Build history of the part. All positions in model axes, mm. Give positions to 0.01 mm unless a question says otherwise; leave off trailing zeros. Order: outer loops, then holes, each group sorted by start corner. A loop starts at its lowest first (then second) coordinate and runs counter-clockwise, first axis right, second up. Notation, with made-up numbers: M -15.75,73.5 L 7.25,73.5 A19 cw 7.25,82.5 Z; hole C 15,69 d10. An arc over 180 degrees is marked long. One line per item, written item: value. Start each with the question number.
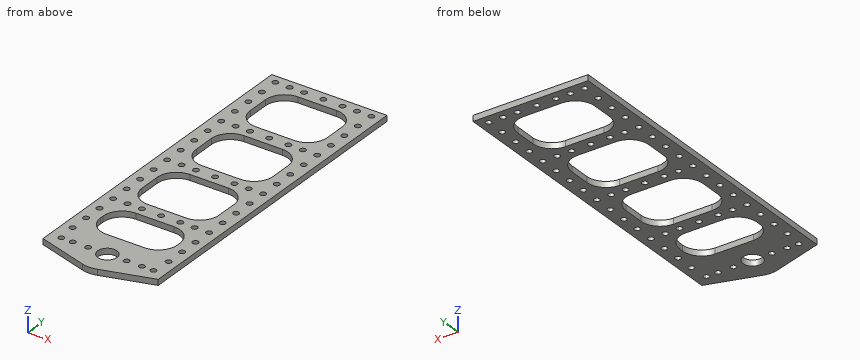
from build123d import *

# Parameters (mm, degrees)
SKETCH1_W           = 40
SKETCH1_H           = 31.068216144
SKETCH1_R           = 1.5
SKETCH1_H_2         = 21.795351568
SKETCH1_R_2         = 5
BOSS_EXTRUDE1_DEPTH = 3
FILLET1_R           = 10


with BuildPart() as part:
    # Sketch1 → Boss-Extrude1 (new body)
    with BuildSketch(Plane.XY):
        with BuildLine():
            Line((-29.546509682, -3.213846621), (-3.468555942, -11.131569065))
            ThreePointArc((-3.468555942, -11.131569065), (0.453490318, -11.713846621), (4.375536577, -11.131569065))
            Line((4.375536577, -11.131569065), (30.453490318, -3.213846621))
            Line((30.453490318, -3.213846621), (30.453490318, 166.286153379))
            Line((30.453490318, 166.286153379), (-29.546509682, 166.286153379))
            Line((-29.546509682, 166.286153379), (-29.546509682, -3.213846621))
        make_face()
        with Locations((0.453490318, 141.752045307)):
            Rectangle(SKETCH1_W, SKETCH1_H, mode=Mode.SUBTRACT)
        with Locations((0.453490318, 101.683829163)):
            Rectangle(SKETCH1_W, SKETCH1_H, mode=Mode.SUBTRACT)
        with Locations((0.453490318, 121.717937235)):
            Circle(SKETCH1_R, mode=Mode.SUBTRACT)
        with Locations((0.453490318, 61.615613019)):
            Rectangle(SKETCH1_W, SKETCH1_H, mode=Mode.SUBTRACT)
        with Locations((0.453490318, 81.649721091)):
            Circle(SKETCH1_R, mode=Mode.SUBTRACT)
        with Locations((0.453490318, 26.183829163)):
            Rectangle(SKETCH1_W, SKETCH1_H_2, mode=Mode.SUBTRACT)
        with Locations((0.453490318, 41.581504947)):
            Circle(SKETCH1_R, mode=Mode.SUBTRACT)
        with Locations((0.453490318, 161.786153379)):
            Circle(SKETCH1_R, mode=Mode.SUBTRACT)
        with Locations((10.453490318, 161.786153379)):
            Circle(SKETCH1_R, mode=Mode.SUBTRACT)
        with Locations((17.953490318, 161.786153379)):
            Circle(SKETCH1_R, mode=Mode.SUBTRACT)
        with Locations((25.453490318, 161.786153379)):
            Circle(SKETCH1_R, mode=Mode.SUBTRACT)
        with Locations((24.453490318, 1.786153379)):
            Circle(SKETCH1_R, mode=Mode.SUBTRACT)
        with Locations((18.453490318, 1.786153379)):
            Circle(SKETCH1_R, mode=Mode.SUBTRACT)
        with Locations((10.453490318, 1.786153379)):
            Circle(SKETCH1_R, mode=Mode.SUBTRACT)
        with Locations((0.453490318, 1.786153379)):
            Circle(SKETCH1_R_2, mode=Mode.SUBTRACT)
        with Locations((-9.546509682, 161.786153379)):
            Circle(SKETCH1_R, mode=Mode.SUBTRACT)
        with Locations((-17.046509682, 161.786153379)):
            Circle(SKETCH1_R, mode=Mode.SUBTRACT)
        with Locations((-24.546509682, 161.786153379)):
            Circle(SKETCH1_R, mode=Mode.SUBTRACT)
        with Locations((-9.546509682, 1.786153379)):
            Circle(SKETCH1_R, mode=Mode.SUBTRACT)
        with Locations((-17.546509682, 1.786153379)):
            Circle(SKETCH1_R, mode=Mode.SUBTRACT)
        with Locations((-23.546509682, 1.786153379)):
            Circle(SKETCH1_R, mode=Mode.SUBTRACT)
        with Locations((-24.546509682, 11.581504947)):
            Circle(SKETCH1_R, mode=Mode.SUBTRACT)
        with Locations((-24.546509682, 21.581504947)):
            Circle(SKETCH1_R, mode=Mode.SUBTRACT)
        with Locations((-24.546509682, 31.581504947)):
            Circle(SKETCH1_R, mode=Mode.SUBTRACT)
        with Locations((-24.546509682, 41.581504947)):
            Circle(SKETCH1_R, mode=Mode.SUBTRACT)
        with Locations((-24.546509682, 51.649721091)):
            Circle(SKETCH1_R, mode=Mode.SUBTRACT)
        with Locations((-24.546509682, 61.649721091)):
            Circle(SKETCH1_R, mode=Mode.SUBTRACT)
        with Locations((-24.546509682, 71.649721091)):
            Circle(SKETCH1_R, mode=Mode.SUBTRACT)
        with Locations((-24.546509682, 81.649721091)):
            Circle(SKETCH1_R, mode=Mode.SUBTRACT)
        with Locations((-24.546509682, 91.717937235)):
            Circle(SKETCH1_R, mode=Mode.SUBTRACT)
        with Locations((-24.546509682, 101.717937235)):
            Circle(SKETCH1_R, mode=Mode.SUBTRACT)
        with Locations((-24.546509682, 111.717937235)):
            Circle(SKETCH1_R, mode=Mode.SUBTRACT)
        with Locations((-24.546509682, 121.717937235)):
            Circle(SKETCH1_R, mode=Mode.SUBTRACT)
        with Locations((-24.546509682, 131.786153379)):
            Circle(SKETCH1_R, mode=Mode.SUBTRACT)
        with Locations((-24.546509682, 141.786153379)):
            Circle(SKETCH1_R, mode=Mode.SUBTRACT)
        with Locations((-24.546509682, 151.786153379)):
            Circle(SKETCH1_R, mode=Mode.SUBTRACT)
        with Locations((25.453490318, 111.717937235)):
            Circle(SKETCH1_R, mode=Mode.SUBTRACT)
        with Locations((25.453490318, 151.786153379)):
            Circle(SKETCH1_R, mode=Mode.SUBTRACT)
        with Locations((25.453490318, 141.786153379)):
            Circle(SKETCH1_R, mode=Mode.SUBTRACT)
        with Locations((25.453490318, 131.786153379)):
            Circle(SKETCH1_R, mode=Mode.SUBTRACT)
        with Locations((25.453490318, 121.717937235)):
            Circle(SKETCH1_R, mode=Mode.SUBTRACT)
        with Locations((25.453490318, 11.581504947)):
            Circle(SKETCH1_R, mode=Mode.SUBTRACT)
        with Locations((25.453490318, 21.581504947)):
            Circle(SKETCH1_R, mode=Mode.SUBTRACT)
        with Locations((25.453490318, 31.581504947)):
            Circle(SKETCH1_R, mode=Mode.SUBTRACT)
        with Locations((25.453490318, 41.581504947)):
            Circle(SKETCH1_R, mode=Mode.SUBTRACT)
        with Locations((25.453490318, 51.649721091)):
            Circle(SKETCH1_R, mode=Mode.SUBTRACT)
        with Locations((25.453490318, 61.649721091)):
            Circle(SKETCH1_R, mode=Mode.SUBTRACT)
        with Locations((25.453490318, 71.649721091)):
            Circle(SKETCH1_R, mode=Mode.SUBTRACT)
        with Locations((25.453490318, 81.649721091)):
            Circle(SKETCH1_R, mode=Mode.SUBTRACT)
        with Locations((25.453490318, 91.717937235)):
            Circle(SKETCH1_R, mode=Mode.SUBTRACT)
        with Locations((25.453490318, 101.717937235)):
            Circle(SKETCH1_R, mode=Mode.SUBTRACT)
        with Locations((-9.546509682, 41.581504947)):
            Circle(SKETCH1_R, mode=Mode.SUBTRACT)
        with Locations((-17.046509682, 41.581504947)):
            Circle(SKETCH1_R, mode=Mode.SUBTRACT)
        with Locations((10.453490318, 41.581504947)):
            Circle(SKETCH1_R, mode=Mode.SUBTRACT)
        with Locations((17.953490318, 41.581504947)):
            Circle(SKETCH1_R, mode=Mode.SUBTRACT)
        with Locations((-9.546509682, 81.649721091)):
            Circle(SKETCH1_R, mode=Mode.SUBTRACT)
        with Locations((-17.046509682, 81.649721091)):
            Circle(SKETCH1_R, mode=Mode.SUBTRACT)
        with Locations((10.453490318, 81.649721091)):
            Circle(SKETCH1_R, mode=Mode.SUBTRACT)
        with Locations((17.953490318, 81.649721091)):
            Circle(SKETCH1_R, mode=Mode.SUBTRACT)
        with Locations((-9.546509682, 121.717937235)):
            Circle(SKETCH1_R, mode=Mode.SUBTRACT)
        with Locations((-17.046509682, 121.717937235)):
            Circle(SKETCH1_R, mode=Mode.SUBTRACT)
        with Locations((17.953490318, 121.717937235)):
            Circle(SKETCH1_R, mode=Mode.SUBTRACT)
        with Locations((10.453490318, 121.717937235)):
            Circle(SKETCH1_R, mode=Mode.SUBTRACT)
    extrude(amount=BOSS_EXTRUDE1_DEPTH)

    # Fillet1
    fillet1_edges = [part.edges().sort_by_distance(p)[0] for p in [
        (20.453490318, 157.286153379, 1.5),
        (-19.546509682, 157.286153379, 1.5),
        (-19.546509682, 126.217937235, 1.5),
        (20.453490318, 126.217937235, 1.5),
        (-19.546509682, 37.081504947, 1.5),
        (-19.546509682, 15.286153379, 1.5),
        (20.453490318, 15.286153379, 1.5),
        (20.453490318, 37.081504947, 1.5),
        (-19.546509682, 77.149721091, 1.5),
        (-19.546509682, 46.081504947, 1.5),
        (20.453490318, 46.081504947, 1.5),
        (20.453490318, 77.149721091, 1.5),
        (-19.546509682, 117.217937235, 1.5),
        (-19.546509682, 86.149721091, 1.5),
        (20.453490318, 86.149721091, 1.5),
        (20.453490318, 117.217937235, 1.5),
    ]]
    fillet(fillet1_edges, radius=FILLET1_R)


solid = part.part
1) Slice it at A-A (x = 14). List the corners of the cut face in (y, z).
2) Drill centre lines: line 1 (Y direction, x = 4, z = 1.6); line 2 (Y direction, x = 19.5, z = 2.4); line 3 (Y direction, x = 12, z = 2.45). Where is each one in solid material? Low to high.
3) Drop flat-ended pins along their axis: P1, Ø4, axis at x = 25.45, y = 101.72, coming from the -Z side; P2, Ø5, axis at x = -15, y = 148, coming from the +Z side; P3, Ø0.9, axis at x = 2, z = 2, coming from the -Y side. Give the stop position or say it passes through.
4) Slice it at B-B (z = 0.6). State how many separate pieces and enclosed holes the cut face has, plus the area to 3 significant figures.
Results list:
1. outline: M -8.21,0 L 15.94,0 L 15.94,3 L -8.21,3 Z; M 36.43,0 L 46.73,0 L 46.73,3 L 36.43,3 Z; M 76.5,0 L 86.8,0 L 86.8,3 L 76.5,3 Z; M 116.57,0 L 126.87,0 L 126.87,3 L 116.57,3 Z; M 156.64,0 L 166.29,0 L 166.29,3 L 156.64,3 Z
2. line 1: y = -11.24 to -1.74, 5.31 to 15.29, 37.08 to 46.08, 77.15 to 86.15, 117.22 to 126.22, 157.29 to 166.29
2. line 2: y = -6.54 to 0.71, 2.86 to 21.02, 31.34 to 51.82, 71.41 to 91.89, 111.48 to 131.96, 151.55 to 166.29
2. line 3: y = -8.82 to 15.41, 36.96 to 46.2, 77.03 to 86.27, 117.1 to 126.34, 157.17 to 166.29
3. P1: stops at z = 0
3. P2: passes through
3. P3: stops at y = -11.67
4. separate pieces: 1
4. enclosed holes: 63
4. area: 5,700 mm²
